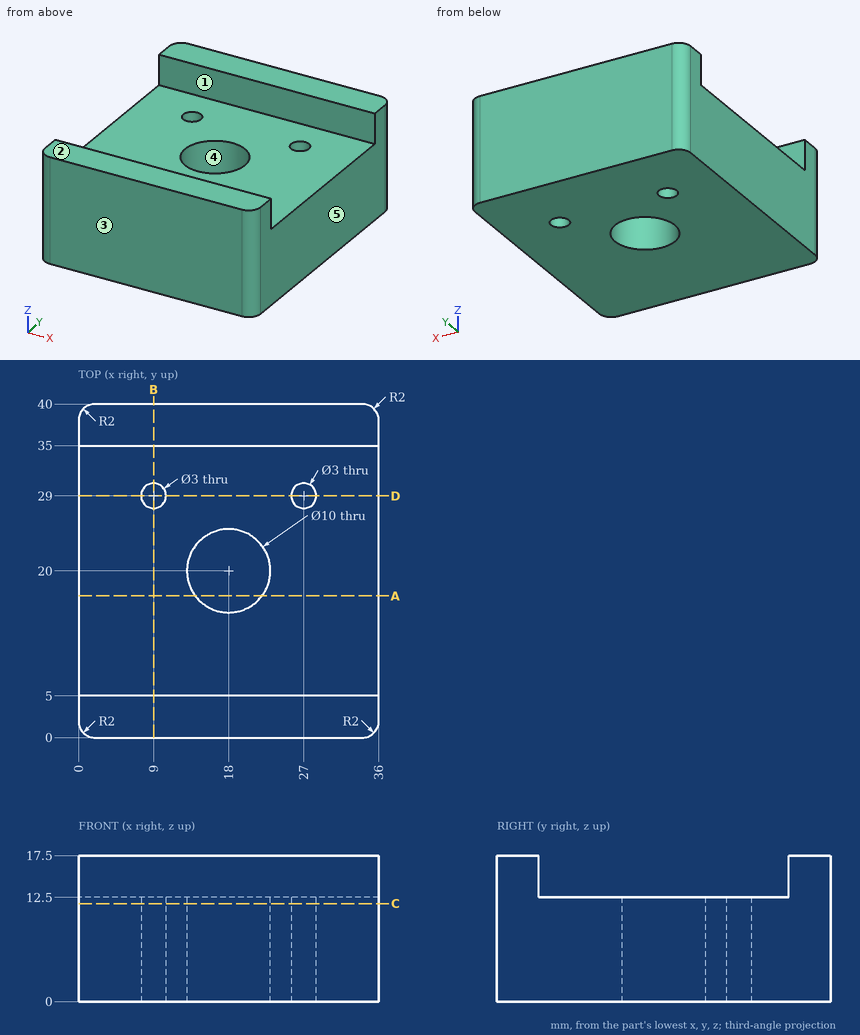
For this review, use the dimensioned drawing (mm, ordinates from the lowest corner) and the shaded views. A direction names the side the tool comes from. Round coordinates to 2 decimals unless told otherwise and drop trailing zeros. Order: outer loops, then holes, each group sorted by start corner. A loop starts at its lowest first (then second) coordinate and runs counter-clockwise, first axis right, second up. Notation, with made-up numbers: (67.25, -17.5) -> (95.25, -17.5) arc R14 ccw to (95.25, 7.5) -> close; hole circle Ø7 at (12, 54.25). An arc over 180 degrees is marked (long way). One line per item, written item: value. Start each with the question number.
Q1. Take a section at C-C (z = 11.75). Write out the cut boundary in (x, y), and give its area (3 significant figures).
Q2. Mouldability with a two-part tool opening along Y and no side actions: class the marked faces 3, 4 and 5 as released by +Y, released by -Y, zero draft, split by the parting line, or undercut.
Q3. Take a section at A-A (y = 17). Write out the cut boundary in (x, z), and give its area (3 significant figures).
Q4. Clearance check with a flat-ended pin moving along its axis: pin 1 Ø12 at (x, y) = (6, 14.5) entering from +Z. State where the tip first meets the part, or that it passes through.
Q5. Take a section at B-B (x = 9). Write out the cut boundary in (y, z), and give its area (4 significant figures).
Q6. Wall thickness on line 1 (Y direction, x = 18, z = 3.5); line 2 (Y direction, x = 22, z = 14.5); line 3 (Z direction, x = 15.5, y = 12): over which ranges is each line inside the solid? List them lowest first.
Q7. Machinability: for the marked faces 1 and 2, which of the approach directions +Z, -Z, +X, -X, +Y, -Y give a long, thin tool a straight path to every point of the face, cutting with its end or side? Answer none if there is none.
Q8. Take a section at D-D (y = 29). Write out the cut boundary in (x, z), and give its area (3 significant figures).
Reported:
1. outline: (0, 2) arc R2 ccw to (2, 0) -> (34, 0) arc R2 ccw to (36, 2) -> (36, 38) arc R2 ccw to (34, 40) -> (2, 40) arc R2 ccw to (0, 38) -> close; hole circle Ø3 at (9, 29); hole circle Ø10 at (18, 20); hole circle Ø3 at (27, 29)
1. area: 1,340 mm2
2. face 3: released by -Y
2. face 4: undercut
2. face 5: zero draft
3. outline: (0, 0) -> (14, 0) -> (14, 12.5) -> (0, 12.5) -> close; (22, 0) -> (36, 0) -> (36, 12.5) -> (22, 12.5) -> close
3. area: 350 mm2
4. pin 1: stops at z = 12.5
5. outline: (0, 0) -> (27.5, 0) -> (27.5, 12.5) -> (5, 12.5) -> (5, 17.5) -> (0, 17.5) -> close; (30.5, 0) -> (40, 0) -> (40, 17.5) -> (35, 17.5) -> (35, 12.5) -> (30.5, 12.5) -> close
5. area: 512.5 mm2
6. line 1: y = 0 to 15, 25 to 40
6. line 2: y = 0 to 5, 35 to 40
6. line 3: z = 0 to 12.5
7. face 1: +Z, +X, -X
7. face 2: +Z, +X, -X, +Y, -Y
8. outline: (0, 0) -> (7.5, 0) -> (7.5, 12.5) -> (0, 12.5) -> close; (10.5, 0) -> (25.5, 0) -> (25.5, 12.5) -> (10.5, 12.5) -> close; (28.5, 0) -> (36, 0) -> (36, 12.5) -> (28.5, 12.5) -> close
8. area: 375 mm2
